```python
from build123d import *

# Parameters (mm, degrees)
BOSS_EXTRUDE1_DEPTH         = 12.7
SKETCH2_W                   = 852.307145123
SKETCH2_H                   = 152.4
CUT_EXTRUDE1_DEPTH          = 12.7
CUT_EXTRUDE2_DEPTH          = 12.7
F_1_4_0_25_DIAMETER_HOLE1_D = 6.35
CUT_EXTRUDE3_DEPTH          = 13.7


with BuildPart() as part:
    # Sketch1 → Boss-Extrude1 (new body)
    with BuildSketch(Plane(origin=(0, 0, 0), x_dir=(0, 0, -1), z_dir=(1, 0, 0))):
        with BuildLine():
            Line((0, 609.6), (323.85, 609.6))
            Line((323.85, 609.6), (323.85, 0))
            Line((323.85, 0), (0, 0))
            Line((0, 0), (0, 31.75))
            ThreePointArc((0, 31.75), (188.340145046, 304.8), (0, 577.85))
            Line((0, 577.85), (0, 609.6))
        make_face()
    extrude(amount=BOSS_EXTRUDE1_DEPTH)

    # Sketch2 → Cut-Extrude1 (cut)
    with BuildSketch(Plane(origin=(12.7, 0, 0), x_dir=(0, 0, -1), z_dir=(1, 0, 0))):
        with Locations((192.653341095, 76.2)):
            Rectangle(SKETCH2_W, SKETCH2_H)
    extrude(amount=-CUT_EXTRUDE1_DEPTH, mode=Mode.SUBTRACT)

    # Sketch3 → Cut-Extrude2 (cut)
    with BuildSketch(Plane(origin=(12.7, 0, 0), x_dir=(0, 0, -1), z_dir=(1, 0, 0))):
        with BuildLine():
            Line((270.760801555, 152.4), (323.85, 152.4))
            Line((323.85, 152.4), (323.85, 609.6))
            Line((323.85, 609.6), (161.925, 609.6))
            ThreePointArc((161.925, 609.6), (289.589524386, 398.436253262), (270.760801555, 152.4))
        make_face()
    extrude(amount=-CUT_EXTRUDE2_DEPTH, mode=Mode.SUBTRACT)

    # 1/4 (0.25) Diameter Hole1 (through all)
    with Locations(Plane(origin=(12.7, 0, 0), x_dir=(0, 0, -1), z_dir=(1, 0, 0))):
        with Locations((181.354437919, 165.1), (191.91696262, 189.121698017), (200.459714845, 213.933596133), (206.924338933, 239.366203925), (211.266674948, 265.245790893), (213.457060331, 291.395573216), (213.480532529, 317.636921367), (211.336931202, 343.790580328), (207.040899322, 369.677894089), (200.621783143, 395.122026048), (192.123431737, 419.949166985), (181.603897461, 443.989722351), (169.1350394, 467.079470776), (154.8020325, 489.060685868), (138.70278573, 509.783213636), (120.94727327, 529.105498206), (101.656783275, 546.89554878), (80.96308935, 563.031841274), (59.00755041, 577.404148448), (35.940145046, 589.914292872)):
            Hole(F_1_4_0_25_DIAMETER_HOLE1_D / 2)

    # Sketch6 → Cut-Extrude3 (cut, through all)
    with BuildSketch(Plane(origin=(12.7, 0, 0), x_dir=(0, 0, -1), z_dir=(1, 0, 0))):
        with BuildLine():
            Line((161.925, 609.6), (114.092348386, 609.6))
            ThreePointArc((114.092348386, 609.6), (257.747151872, 403.163135962), (238.492774693, 152.4))
            Line((238.492774693, 152.4), (270.760801555, 152.4))
            ThreePointArc((270.760801555, 152.4), (289.589524386, 398.436253262), (161.925, 609.6))
        make_face()
    extrude(amount=-CUT_EXTRUDE3_DEPTH, mode=Mode.SUBTRACT)


solid = part.part
```
Part model, mm, in its own coordinate system. Round coordinates to 2 decimals unless told otherwise and drop trailing zeros. Loops run counter-clockwise (first coordinate to the right, second up) from the corner with the lowest first, then second, coordinate; pieces in that order, holes last. Notation, with made-up numbers: (55.5, 6) -> (108.5, 6) arc R27 ccw to (108.5, 36) -> close; hole circle Ø3 at (13, 72.25). An arc over 180 degrees is marked (long way). Use one line per item in the form item = value. Start each with the question number.
Item 1: Band-saw the part on A-A (x = 8.5). Give the number of separate pieces and of enclosed holes in the cut face, plus the area to 3 significant figures.
Item 2: Two-plate mould, pull along Y, no slides. Class faces 1 (the cylindrical face through (6.261, 395.876, -173.779)), 2 (the cylindrical face through (6.44, 406.62, -256.79)), 3 (the flat face through (6, 152.4, -191)), 4 (the flat face through (6, 609.6, -56)): released by +Y, released by -Y, zero draft, split by the parting line, or undercut.
Item 3: Drop flat-ended pins along their axis: pin 1 Ø5 at (y, z) = (165.1, -181.35) entering from +X; pin 2 Ø1 at (x, y) = (7, 418) entering from +Z; pin 3 Ø3 at (x, y) = (10.5, 538) entering from +Z; pin 4 Ø1.5 at (x, y) = (4.5, 224.5) entering from -Z. Give the stop position or say it passes through.
Item 4: Drill centre lines: line 1 along Y through (x, z) = (2.75, -194); line 2 along Y through (x, z) = (10, -199); line 3 along Z through (x, y) = (3.25, 584.5). Where is each one in solid material? Low to high.
Item 5: Band-saw the part on B-B (z = -129.5). List the corners of the cut face in (x, y).
Data:
q1.separate_pieces = 1
q1.enclosed_holes = 20
q1.area = 43,400 mm^2
q2.face_1 = undercut
q2.face_2 = split by the parting line
q2.face_3 = released by -Y
q2.face_4 = released by +Y
q3.pin_1 = through
q3.pin_2 = -165.3
q3.pin_3 = -70.13
q3.pin_4 = -262.35
q4.line_1 = 152.4 to 186.73, 191.52 to 417.39, 422.51 to 532.18
q4.line_2 = 152.4 to 211.11, 216.75 to 392.39, 397.85 to 525.48
q4.line_3 = -145.5 to 0
q5.outline = (0, 480.62) -> (12.7, 480.62) -> (12.7, 597.98) -> (0, 597.98) -> close
